from build123d import *

# Parameters (mm, degrees)
SKETCH2_R           = 88.9
BOSS_EXTRUDE1_DEPTH = 76.2
FILLET1_R           = 25.4
SHELL1_T            = -6.35
CUT_EXTRUDE1_REACH  = 145.824
SKETCH6_R           = 31.75
BOSS_EXTRUDE2_DEPTH = 19.05
CUT_EXTRUDE2_REACH  = 155.979
SKETCH7_R           = 19.05
BOSS_EXTRUDE3_START = -12.7
SKETCH9_R           = 9.525
BOSS_EXTRUDE3_DEPTH = 12.7
CIRPATTERN1_COUNT   = 3


with BuildPart() as part:
    # Sketch2 → Boss-Extrude1 (new body)
    with BuildSketch(Plane(origin=(0, 0, 0), x_dir=(1, 0, 0), z_dir=(0, 1, 0))):
        with Locations(Location((0, 0, 0), (0, 0, 90))):
            Circle(SKETCH2_R)
    extrude(amount=BOSS_EXTRUDE1_DEPTH)

    # Fillet1
    fillet1_edges = [part.edges().sort_by_distance(p)[0] for p in [
        (0, 0, 88.9),
    ]]
    fillet(fillet1_edges, radius=FILLET1_R)

    # Shell1
    shell1_openings = [part.faces().sort_by_distance(p)[0] for p in [
        (0, 76.2, 0),
    ]]
    offset(amount=SHELL1_T, openings=shell1_openings, kind=Kind.INTERSECTION)

    # Sketch3 → Cut-Extrude1 (cut, up to next)
    with BuildSketch(Plane(origin=(0, 6.35, 0), x_dir=(1, 0, 0), z_dir=(0, 1, 0)), mode=Mode.PRIVATE) as cut_extrude1_sk1:
        with BuildLine():
            Line((50.165, 50.699645362), (50.165, -50.900354638))
            ThreePointArc((50.165, -50.900354638), (45.72, -55.345354638), (41.275, -50.900354638))
            Line((41.275, -50.900354638), (41.275, 50.699645362))
            ThreePointArc((41.275, 50.699645362), (45.72, 55.144645362), (50.165, 50.699645362))
        make_face()
    cut_extrude1_tool1 = extrude(cut_extrude1_sk1.sketch, amount=-CUT_EXTRUDE1_REACH, mode=Mode.PRIVATE) & part.part
    # Sketch3 → Cut-Extrude1 (cut, up to next)
    with BuildSketch(Plane(origin=(0, 6.35, 0), x_dir=(1, 0, 0), z_dir=(0, 1, 0)), mode=Mode.PRIVATE) as cut_extrude1_sk2:
        with BuildLine():
            Line((26.035, 50.699645362), (26.035, -50.900354638))
            ThreePointArc((26.035, -50.900354638), (30.48, -55.345354638), (34.925, -50.900354638))
            Line((34.925, -50.900354638), (34.925, 50.699645362))
            ThreePointArc((34.925, 50.699645362), (30.48, 55.144645362), (26.035, 50.699645362))
        make_face()
    cut_extrude1_tool2 = extrude(cut_extrude1_sk2.sketch, amount=-CUT_EXTRUDE1_REACH, mode=Mode.PRIVATE) & part.part
    # Sketch3 → Cut-Extrude1 (cut, up to next)
    with BuildSketch(Plane(origin=(0, 6.35, 0), x_dir=(1, 0, 0), z_dir=(0, 1, 0)), mode=Mode.PRIVATE) as cut_extrude1_sk3:
        with BuildLine():
            Line((10.795, 50.699645362), (10.795, -50.900354638))
            ThreePointArc((10.795, -50.900354638), (15.24, -55.345354638), (19.685, -50.900354638))
            Line((19.685, -50.900354638), (19.685, 50.699645362))
            ThreePointArc((19.685, 50.699645362), (15.24, 55.144645362), (10.795, 50.699645362))
        make_face()
    cut_extrude1_tool3 = extrude(cut_extrude1_sk3.sketch, amount=-CUT_EXTRUDE1_REACH, mode=Mode.PRIVATE) & part.part
    # Sketch3 → Cut-Extrude1 (cut, up to next)
    with BuildSketch(Plane(origin=(0, 6.35, 0), x_dir=(1, 0, 0), z_dir=(0, 1, 0)), mode=Mode.PRIVATE) as cut_extrude1_sk4:
        with BuildLine():
            Line((-4.445, 50.699645362), (-4.445, -50.900354638))
            ThreePointArc((-4.445, -50.900354638), (0, -55.345354638), (4.445, -50.900354638))
            Line((4.445, -50.900354638), (4.445, 50.699645362))
            ThreePointArc((4.445, 50.699645362), (0, 55.144645362), (-4.445, 50.699645362))
        make_face()
    cut_extrude1_tool4 = extrude(cut_extrude1_sk4.sketch, amount=-CUT_EXTRUDE1_REACH, mode=Mode.PRIVATE) & part.part
    # Sketch3 → Cut-Extrude1 (cut, up to next)
    with BuildSketch(Plane(origin=(0, 6.35, 0), x_dir=(1, 0, 0), z_dir=(0, 1, 0)), mode=Mode.PRIVATE) as cut_extrude1_sk5:
        with BuildLine():
            Line((-19.685, 50.699645362), (-19.685, -50.900354638))
            ThreePointArc((-19.685, -50.900354638), (-15.24, -55.345354638), (-10.795, -50.900354638))
            Line((-10.795, -50.900354638), (-10.795, 50.699645362))
            ThreePointArc((-10.795, 50.699645362), (-15.24, 55.144645362), (-19.685, 50.699645362))
        make_face()
    cut_extrude1_tool5 = extrude(cut_extrude1_sk5.sketch, amount=-CUT_EXTRUDE1_REACH, mode=Mode.PRIVATE) & part.part
    # Sketch3 → Cut-Extrude1 (cut, up to next)
    with BuildSketch(Plane(origin=(0, 6.35, 0), x_dir=(1, 0, 0), z_dir=(0, 1, 0)), mode=Mode.PRIVATE) as cut_extrude1_sk6:
        with BuildLine():
            Line((-34.925, 50.699645362), (-34.925, -50.900354638))
            ThreePointArc((-34.925, -50.900354638), (-30.48, -55.345354638), (-26.035, -50.900354638))
            Line((-26.035, -50.900354638), (-26.035, 50.699645362))
            ThreePointArc((-26.035, 50.699645362), (-30.48, 55.144645362), (-34.925, 50.699645362))
        make_face()
    cut_extrude1_tool6 = extrude(cut_extrude1_sk6.sketch, amount=-CUT_EXTRUDE1_REACH, mode=Mode.PRIVATE) & part.part
    # Sketch3 → Cut-Extrude1 (cut, up to next)
    with BuildSketch(Plane(origin=(0, 6.35, 0), x_dir=(1, 0, 0), z_dir=(0, 1, 0)), mode=Mode.PRIVATE) as cut_extrude1_sk7:
        with BuildLine():
            Line((-50.165, 50.699645362), (-50.165, -50.900354638))
            ThreePointArc((-50.165, -50.900354638), (-45.72, -55.345354638), (-41.275, -50.900354638))
            Line((-41.275, -50.900354638), (-41.275, 50.699645362))
            ThreePointArc((-41.275, 50.699645362), (-45.72, 55.144645362), (-50.165, 50.699645362))
        make_face()
    cut_extrude1_tool7 = extrude(cut_extrude1_sk7.sketch, amount=-CUT_EXTRUDE1_REACH, mode=Mode.PRIVATE) & part.part
    add(cut_extrude1_tool1.solids().sort_by_distance((45.72, 6.35, 0.100355))[0], mode=Mode.SUBTRACT)
    add(cut_extrude1_tool2.solids().sort_by_distance((30.48, 6.35, 0.100355))[0], mode=Mode.SUBTRACT)
    add(cut_extrude1_tool3.solids().sort_by_distance((15.24, 6.35, 0.100355))[0], mode=Mode.SUBTRACT)
    add(cut_extrude1_tool4.solids().sort_by_distance((0, 6.35, 0.100355))[0], mode=Mode.SUBTRACT)
    add(cut_extrude1_tool5.solids().sort_by_distance((-15.24, 6.35, 0.100355))[0], mode=Mode.SUBTRACT)
    add(cut_extrude1_tool6.solids().sort_by_distance((-30.48, 6.35, 0.100355))[0], mode=Mode.SUBTRACT)
    add(cut_extrude1_tool7.solids().sort_by_distance((-45.72, 6.35, 0.100355))[0], mode=Mode.SUBTRACT)

    # Sketch6 → Boss-Extrude2 (add)
    with BuildSketch(Plane(origin=(0, 6.35, 0), x_dir=(1, 0, 0), z_dir=(0, 1, 0))):
        with Locations(Location((0, 0, 0), (0, 0, 270))):
            Circle(SKETCH6_R)
    extrude(amount=-BOSS_EXTRUDE2_DEPTH)

    # Sketch7 → Cut-Extrude2 (cut, up to next)
    with BuildSketch(Plane.XZ.offset(12.7), mode=Mode.PRIVATE) as cut_extrude2_sk1:
        with Locations(Location((0, 0, 0), (0, 0, 270))):
            Circle(SKETCH7_R)
    cut_extrude2_tool1 = extrude(cut_extrude2_sk1.sketch, amount=-CUT_EXTRUDE2_REACH, mode=Mode.PRIVATE) & part.part
    add(cut_extrude2_tool1.solids().sort_by_distance((0, -12.7, 0))[0], mode=Mode.SUBTRACT)

    # Sketch9 → Boss-Extrude3 (add)
    with BuildSketch(Plane(origin=(0, 76.2, 0), x_dir=(1, 0, 0), z_dir=(0, 1, 0)).offset(BOSS_EXTRUDE3_START)):
        with BuildLine():
            Line((-19.05, 107.95), (-19.05, 86.834944003))
            ThreePointArc((-19.05, 86.834944003), (0, 88.9), (19.05, 86.834944003))
            Line((19.05, 86.834944003), (19.05, 107.95))
            ThreePointArc((19.05, 107.95), (0, 127), (-19.05, 107.95))
        make_face()
        with Locations(Location((0, 107.95, 0), (0, 0, 270))):
            Circle(SKETCH9_R, mode=Mode.SUBTRACT)
    boss_extrude3 = extrude(amount=BOSS_EXTRUDE3_DEPTH)

    # CirPattern1: Boss-Extrude3 ×3 about axis
    cirpattern1_axis = Axis((0, 0, 0), (0, 1, 0))
    for i in range(1, CIRPATTERN1_COUNT):
        add(boss_extrude3.rotate(cirpattern1_axis, i * 360 / CIRPATTERN1_COUNT))


solid = part.part
Geometry: final body of the model. Coordinates: model frame, mm. A direction names the side the tool comes from. Round coordinates to 2 decimals unless told otherwise and drop trailing zeros. Write each loop counter-clockwise with the first axis right and the second up, starting at its lowest first coordinate (ties: lowest second). Pieces come first, ordered by that corner, then holes. Notation, with made-up numbers: M 13,-8 L 29,-8 A10 cw 29,1 Z; hole C 13.5,68 d9. An arc over 180 degrees is marked long. Write item = value, one per line.
Item 1: Section query C-C on y = 49. Return loops of the section in (x, z).
Findings:
outline = C 0,0 d177.8; hole C 0,0 d165.1
Item 2: Pin query (flat end, axial travel): P1, Ø1.8, axis at x = -33, z = 54.5, coming from the -Y side; P2, Ø1, axis at y = -1.5, z = -2.5, coming from the -X side; P3, Ø6.5, axis at x = 57.5, z = -16, coming from the +Y side. Return the tip coordinate at first contact, or that it passes through.
Findings:
P1 = 0
P2 = -31.69
P3 = 6.35
Item 3: Section query A-A on z = 0. State how many separate pieces and enclosed holes the cut face has, then the cut area to 3 significant figures.
Findings:
separate_pieces = 6
enclosed_holes = 0
area = 1,820 mm^2
Item 4: Pull-direction query (Z, two-part tool) for faces 3 (the face through (-110.191, 69.761, 63.135)), 4 (the face through (55, 0, 1)), 5 (the face through (-30.578, 3.219, 55.344)); classes: pulls with the +Z half, pulls with the -Z half, needs draft (parallel to the pull), parting line crosses it, or undercut.
Findings:
face_3 = parting line crosses it
face_4 = needs draft
face_5 = undercut
Item 5: Material intervals for line 1 along X through (y, z) = (42, 0); line 2 along Z through (x, y) = (-2, 54); line 3 along Y through (x, z) = (38, 21.5), sorted ascending. Write a range as [from, to].
Findings:
line_1 = [-88.9, -82.55], [82.55, 88.9]
line_2 = [-88.88, -82.53], [82.53, 88.88]
line_3 = [0, 6.35]
Item 6: Access query for faces 1 (the face through (-81.848, 50.444, 10.746)), 2 (the face through (50.165, 3, -1)). Directions: +Z, -Z, +X, -X, +Y, -Y. A direction counts if a zero-diameter tool reaches every point of the face in a straight line with its end or side. Return the directions, or none.
Findings:
face_1 = +Y
face_2 = -Y
Item 7: Section query B-B on z = -112. Return loops of the section in (x, y).
Findings:
outline = M -18.61,63.5 L -8.62,63.5 L -8.62,76.2 L -18.61,76.2 Z; M 8.62,63.5 L 18.61,63.5 L 18.61,76.2 L 8.62,76.2 Z
